Read the model definition and answer for the solid it produces. Units are mm, in the model's axes. A direction names the side the tool comes from. Round coordinates to 2 decimals unless told otherwise and drop trailing zeros. Write each loop counter-clockwise with the first axis right and the second up, starting at its lowest first coordinate (ties: lowest second). Pieces come first, ordered by that corner, then holes. Notation, with made-up numbers: (80, 10.5) -> (110, 10.5) arc R35 cw to (110, 43.5) -> close; hole circle Ø3 at (0.25, 25). An arc over 180 degrees is marked (long way). Return JSON: item names as keys, results as strings. Group by question number.
(1) A cutting plane is placed at B-B on x = 9.5. Give the vertices of the cut face in (y, z), then the cut area to 3 significant figures.
(2) A cutting plane is placed at D-D on z = 34. Give the vertices of the cut face in (x, y), then the cut area to 3 significant figures.
(3) A cutting plane is placed at A-A on z = -21.5. Give the vertices of the cut face in (x, y), then the cut area to 3 significant figures.
(4) A cutting plane is placed at C-C on z = 10.75. Give the vertices of the cut face in (x, y), then the cut area to 3 significant figures.
(5) For faces 4 (the flat face through (-25, 3.5, -1)), 5 (the cylindrical face through (-48.794, 49.93, 25.379)), determine the directions among +Z, -Z, +X, -X, +Y, -Y from which every point of the face is accessible in a straight line to the end or side of a thin tool.
(6) Straight lines are drawn through the part: line 1 (X direction, y = 51, z = 0); line 2 (Y direction, x = 39.5, z = 9); line 3 (X direction, y = 1, z = 10.75). For each, find the intervals that lie inside material, in ascending order.
(7) Given pin 1 (3 mm diameter, centred on x = 22.5, z = 0.5, fed in from -Y); pin 2 (4 mm diameter, centred on x = -23.01, z = 0, fed in from +Y); pin 3 (2 mm diameter, centred on x = -2, y = 18.5, fed in from -Z), each flat-ended and moving along its own axis, determine where each tip first touches the part or whether it passes through.
(8) The mould has two halves that part along Z. Classify faces 1 (the flat face through (-10, 5, 10)), 2 (the cylindrical face through (15.02, 2.46, 47.69)), 3 (the flat face through (-25.6, 1.73, 1.52)): released by +Z, released by -Z, zero draft, split by the parting line, or undercut.
```python
from build123d import *

# Parameters (mm, degrees)
SKETCH1_R           = 50
SKETCH1_R_2         = 13.5
SKETCH1_R_3         = 2.65
SKETCH1_R_4         = 1.65
BOSS_EXTRUDE1_DEPTH = 5
SKETCH3_R           = 7.5
BOSS_EXTRUDE2_DEPTH = 40
SKETCH4_R           = 55
SKETCH4_R_2         = 30
BOSS_EXTRUDE3_DEPTH = 10
CUT_EXTRUDE1_DEPTH  = 3.5


with BuildPart() as part:
    # Sketch1 → Boss-Extrude1 (new body)
    with BuildSketch(Plane(origin=(0, 0, 0), x_dir=(1, 0, 0), z_dir=(0, 1, 0))):
        with Locations(Location((0, 0, 0), (0, 0, 270))):
            Circle(SKETCH1_R)
        with Locations(Location((0, 0, 0), (0, 0, 270))):
            Circle(SKETCH1_R_2, mode=Mode.SUBTRACT)
        with Locations(Location((0, 21.5, 0), (0, 0, 270))):
            Circle(SKETCH1_R_3, mode=Mode.SUBTRACT)
        with Locations(Location((23.0125, 0, 0), (0, 0, 270))):
            Circle(SKETCH1_R_4, mode=Mode.SUBTRACT)
        with Locations(Location((-23.0125, 0, 0), (0, 0, 270))):
            Circle(SKETCH1_R_4, mode=Mode.SUBTRACT)
        with Locations(Location((18.619546181, -10.75, 0), (0, 0, 270))):
            Circle(SKETCH1_R_3, mode=Mode.SUBTRACT)
        with Locations(Location((-18.619546181, -10.75, 0), (0, 0, 270))):
            Circle(SKETCH1_R_3, mode=Mode.SUBTRACT)
    extrude(amount=BOSS_EXTRUDE1_DEPTH)

    # Sketch3 → Boss-Extrude2 (add)
    with BuildSketch(Plane(origin=(0, 5, 0), x_dir=(1, 0, 0), z_dir=(0, 1, 0))):
        with Locations(Location((0, 42.5, 0), (0, 0, 89.99967908))):
            Circle(SKETCH3_R)
        with Locations(Location((36.806079661, -21.25, 0), (0, 0, 329.999669783))):
            Circle(SKETCH3_R)
        with Locations(Location((-36.806079661, -21.25, 0), (0, 0, 209.999673972))):
            Circle(SKETCH3_R)
    extrude(amount=BOSS_EXTRUDE2_DEPTH)

    # Sketch4 → Boss-Extrude3 (add)
    with BuildSketch(Plane(origin=(0, 45, 0), x_dir=(1, 0, 0), z_dir=(0, 1, 0))):
        with Locations(Location((0, 0, 0), (0, 0, 270))):
            Circle(SKETCH4_R)
        with Locations(Location((0, 0, 0), (0, 0, 270))):
            Circle(SKETCH4_R_2, mode=Mode.SUBTRACT)
    extrude(amount=BOSS_EXTRUDE3_DEPTH)

    # Sketch5 → Cut-Extrude1 (cut)
    with BuildSketch(Plane(origin=(0, 0, 0), x_dir=(-1, 0, 0), z_dir=(0, -1, 0))):
        Polygon((-26.476601615, 0), (-24.744550808, -3), (-21.280449192, -3), (-19.548398385, 0), (-21.280449192, 3), (-24.744550808, 3), align=None)
        Polygon((26.476601615, 0), (24.744550808, 3), (21.280449192, 3), (19.548398385, 0), (21.280449192, -3), (24.744550808, -3), align=None)
    extrude(amount=-CUT_EXTRUDE1_DEPTH, mode=Mode.SUBTRACT)


solid = part.part
```
Checks:
{
 "1": {"outline": "(0, -49.09) -> (5, -49.09) -> (5, -9.59) -> (0, -9.59) -> close; (0, 9.59) -> (5, 9.59) -> (5, 49.09) -> (0, 49.09) -> close; (45, -54.17) -> (55, -54.17) -> (55, -28.46) -> (45, -28.46) -> close; (45, 28.46) -> (55, 28.46) -> (55, 54.17) -> (45, 54.17) -> close", "area": "909 mm^2"},
 "2": {"outline": "(-43.23, 45) -> (43.23, 45) -> (43.23, 55) -> (-43.23, 55) -> close; (-36.66, 0) -> (36.66, 0) -> (36.66, 5) -> (-36.66, 5) -> close", "area": "1,230 mm^2"},
 "3": {"outline": "(-50.62, 45) -> (-20.92, 45) -> (-20.92, 55) -> (-50.62, 55) -> close; (-45.14, 0) -> (-2.65, 0) -> (-2.65, 5) -> (-45.14, 5) -> close; (2.65, 0) -> (45.14, 0) -> (45.14, 5) -> (2.65, 5) -> close; (20.92, 45) -> (50.62, 45) -> (50.62, 55) -> (20.92, 55) -> close", "area": "1,020 mm^2"},
 "4": {"outline": "(-53.94, 45) -> (-28.01, 45) -> (-28.01, 55) -> (-53.94, 55) -> close; (-48.83, 0) -> (-21.27, 0) -> (-21.27, 5) -> (-48.83, 5) -> close; (-15.97, 0) -> (-8.17, 0) -> (-8.17, 5) -> (-15.97, 5) -> close; (8.17, 0) -> (15.97, 0) -> (15.97, 5) -> (8.17, 5) -> close; (21.27, 0) -> (48.83, 0) -> (48.83, 5) -> (21.27, 5) -> close; (28.01, 45) -> (53.94, 45) -> (53.94, 55) -> (28.01, 55) -> close", "area": "872 mm^2"},
 "5": {"face 4": "-Y", "face 5": "+Y, -Y"},
 "6": {"line 1": "x = -55 to -30, 30 to 55", "line 2": "y = 0 to 5, 45 to 55", "line 3": "x = -48.83 to -21.27, -15.97 to -8.17, 8.17 to 15.97, 21.27 to 48.83"},
 "7": {"pin 1": "stops at y = 3.5", "pin 2": "stops at y = 5", "pin 3": "stops at z = -49.93"},
 "8": {"face 1": "zero draft", "face 2": "split by the parting line", "face 3": "undercut"}
}
